Read the model definition and answer for the solid it produces. Units are mm, in the model's axes. A direction names the side the tool comes from. Coordinates: 2 decimals unless noted, no trailing zeros. Order: outer loops, then holes, each group sorted by start corner. A loop starts at its lowest first (then second) coordinate and runs counter-clockwise, first axis right, second up. Notation, with made-up numbers: M 45,-25.5 L 52,-25.5 A19 cw 52,-19.5 Z; hole C 76.5,1.25 d7. An arc over 180 degrees is marked long. Write each question's results on one line, items separated by ' | '.
```python
from build123d import *

# Parameters (mm, degrees)
SKETCH1_W           = 100.75
SKETCH1_H           = 94
BOSS_EXTRUDE1_DEPTH = 14
SHELL1_T            = -2
SKETCH2_R           = 3.5
SKETCH2_R_2         = 4
BOSS_EXTRUDE2_DEPTH = 6.3
SKETCH3_R           = 1.5
SKETCH3_R_2         = 4
SKETCH3_R_3         = 3.125
SKETCH3_R_4         = 0.75
SKETCH3_W           = 78.75
SKETCH3_H           = 51.25
CUT_EXTRUDE1_DEPTH  = 15
FILLET1_R           = 4.1


with BuildPart() as part:
    # Sketch1 → Boss-Extrude1 (new body)
    with BuildSketch(Plane.XY):
        Rectangle(SKETCH1_W, SKETCH1_H)
    extrude(amount=BOSS_EXTRUDE1_DEPTH)

    # Shell1
    shell1_openings = [part.faces().sort_by_distance(p)[0] for p in [
        (0, 0, 0),
    ]]
    offset(amount=SHELL1_T, openings=shell1_openings, kind=Kind.INTERSECTION)

    # Sketch2 → Boss-Extrude2 (add)
    with BuildSketch(Plane(origin=(0, 0, 12), x_dir=(-1, 0, 0), z_dir=(0, 0, -1))):
        with Locations((-43.975, 40.9)):
            Circle(SKETCH2_R)
        with Locations((-43.975, -24.1)):
            Circle(SKETCH2_R)
        with Locations((43.975, 40.9)):
            Circle(SKETCH2_R)
        with Locations((43.975, -24.1)):
            Circle(SKETCH2_R)
        with Locations((-3.375, -33)):
            Circle(SKETCH2_R_2)
    extrude(amount=BOSS_EXTRUDE2_DEPTH)

    # Sketch3 → Cut-Extrude1 (cut, through all)
    with BuildSketch(Plane.XY.offset(14)):
        with Locations((-44.025, 40.9)):
            Circle(SKETCH3_R)
        with Locations((43.975, 40.9)):
            Circle(SKETCH3_R)
        with Locations((43.975, -24.1)):
            Circle(SKETCH3_R)
        with Locations((-44.025, -24.1)):
            Circle(SKETCH3_R)
        with Locations((36.375, -35.5)):
            Circle(SKETCH3_R_2)
        with Locations((3.375, -33)):
            Circle(SKETCH3_R_3)
        with Locations((19.388263363, -33.242972513)):
            Circle(SKETCH3_R_4)
        with Locations((21.559750082, -34.033329043)):
            Circle(SKETCH3_R_4)
        with Locations((22.715174032, -36.034582029)):
            Circle(SKETCH3_R_4)
        with Locations((22.313899506, -38.310322957)):
            Circle(SKETCH3_R_4)
        with Locations((20.543687313, -39.795707355)):
            Circle(SKETCH3_R_4)
        with Locations((18.232839412, -39.795707355)):
            Circle(SKETCH3_R_4)
        with Locations((16.46262722, -38.310322957)):
            Circle(SKETCH3_R_4)
        with Locations((16.061352693, -36.034582029)):
            Circle(SKETCH3_R_4)
        with Locations((17.216776643, -34.033329043)):
            Circle(SKETCH3_R_4)
        with Locations((19.388263363, -30.927009025)):
            Circle(SKETCH3_R_4)
        with Locations((22.235361921, -31.689886784)):
            Circle(SKETCH3_R_4)
        with Locations((24.319582721, -33.774107583)):
            Circle(SKETCH3_R_4)
        with Locations((25.08246048, -36.621206142)):
            Circle(SKETCH3_R_4)
        with Locations((24.319582721, -39.468304701)):
            Circle(SKETCH3_R_4)
        with Locations((22.235361921, -41.5525255)):
            Circle(SKETCH3_R_4)
        with Locations((19.388263363, -42.31540326)):
            Circle(SKETCH3_R_4)
        with Locations((16.541164804, -41.5525255)):
            Circle(SKETCH3_R_4)
        with Locations((14.456944005, -39.468304701)):
            Circle(SKETCH3_R_4)
        with Locations((13.694066245, -36.621206142)):
            Circle(SKETCH3_R_4)
        with Locations((14.456944005, -33.774107583)):
            Circle(SKETCH3_R_4)
        with Locations((16.541164804, -31.689886784)):
            Circle(SKETCH3_R_4)
        with Locations((0.25, 8.625)):
            Rectangle(SKETCH3_W, SKETCH3_H)
        with BuildLine():
            Line((-24.625, -24), (-14.625, -24))
            ThreePointArc((-14.625, -24), (-13.625, -25), (-14.625, -26))
            Line((-14.625, -26), (-24.625, -26))
            ThreePointArc((-24.625, -26), (-25.625, -25), (-24.625, -24))
        make_face()
        with BuildLine():
            Line((-24.625, -28), (-14.625, -28))
            ThreePointArc((-14.625, -28), (-13.625, -29), (-14.625, -30))
            Line((-14.625, -30), (-24.625, -30))
            ThreePointArc((-24.625, -30), (-25.625, -29), (-24.625, -28))
        make_face()
        with BuildLine():
            Line((-24.625, -32), (-14.625, -32))
            ThreePointArc((-14.625, -32), (-13.625, -33), (-14.625, -34))
            Line((-14.625, -34), (-24.625, -34))
            ThreePointArc((-24.625, -34), (-25.625, -33), (-24.625, -32))
        make_face()
    extrude(amount=-CUT_EXTRUDE1_DEPTH, mode=Mode.SUBTRACT)

    # Fillet1
    fillet1_edges = [part.edges().sort_by_distance(p)[0] for p in [
        (50.375, -47, 7),
        (-50.375, -47, 7),
        (-50.375, 47, 7),
        (50.375, 47, 7),
    ]]
    fillet(fillet1_edges, radius=FILLET1_R)


solid = part.part
```
(1) For faces 1 (the flat face through (6, -35, 5.7)), 2 (the flat face through (-1, 47, 7)), determine the directions among +Z, -Z, +X, -X, +Y, -Y from which every point of the face is accessible in a straight line to the end or side of a thin tool.
Conclusion:
face 1: -Z | face 2: +Z, -Z, +X, -X, +Y
(2) The part is cut by section A-A, the plane z = 9.5. Count the separate pieces of the cut face and the enclosed holes in it, then the cut area to 3 significant figures.
Conclusion:
separate pieces: 6 | enclosed holes: 6 | area: 894 mm²
(3) The mould has two halves that part along X. Classify faces 3 (the flat face through (-48.375, -1, 6)), 4 (the cylindrical face through (-49.206, 45.767, 7.098)), 5 (the flat face through (-1, -47, 7)), 6 (the flat face through (44, -26, 5.7)): pulls with the +X half, pulls with the -X half, needs draft (parallel to the pull), parting line crosses it, or undercut.
Conclusion:
face 3: undercut | face 4: pulls with the -X half | face 5: needs draft | face 6: undercut
(4) Given pin 1 (1.2 mm diameter, centred on x = 16.54, y = -41.55, fed in from -Z); pin 2 (2.5 mm diameter, centred on x = 24.32, y = -39.47, fed in from -Z), each flat-ended and moving along its own axis, determine where each tip first touches the part or whether it passes through.
Conclusion:
pin 1: through | pin 2: z = 12
(5) The part is cut by section B-B, the plane y = 9. Write down the section's boundary in (x, z) (3 decimals).
Conclusion:
outline: M -50.375,0 L -48.375,0 L -48.375,12 L -39.125,12 L -39.125,14 L -50.375,14 Z; M 39.625,12 L 48.375,12 L 48.375,0 L 50.375,0 L 50.375,14 L 39.625,14 Z
(6) The part is cut by section C-C, the plane x = 10.5. Write down the section's boundary in (y, z).
Conclusion:
outline: M -47,0 L -45,0 L -45,12 L -17,12 L -17,14 L -47,14 Z; M 34.25,12 L 45,12 L 45,0 L 47,0 L 47,14 L 34.25,14 Z
(7) The part is cut by section D-D, the plane y = 40.9. Write down the section's boundary in (x, z) (3 decimals), then the cut area to 3 significant figures.
Conclusion:
outline: M -50.375,0 L -48.375,0 L -48.375,12 L -47.475,12 L -47.475,5.7 L -45.525,5.7 L -45.525,14 L -50.375,14 Z; M -42.525,5.7 L -40.475,5.7 L -40.475,12 L 40.475,12 L 40.475,5.7 L 42.475,5.7 L 42.475,14 L -42.525,14 Z; M 45.475,5.7 L 47.475,5.7 L 47.475,12 L 48.375,12 L 48.375,0 L 50.375,0 L 50.375,14 L 45.475,14 Z | area: 288 mm²
(8) Straight lines are drawn through the part: line 1 (Y direction, x = 36, z = 13); line 2 (X direction, y = -11, z = 12.5) (3 decimals); line 3 (X direction, y = 31, z = 6) (3 decimals). For each, find the intervals that lie inside material, in ascending order.
Conclusion:
line 1: -47 to -39.48, -31.52 to -17, 34.25 to 47 | line 2: -50.375 to -39.125, 39.625 to 50.375 | line 3: -50.375 to -48.375, 48.375 to 50.375
